Drawing for the job (mm, zero at the part's lowest x, y, z). A direction names the side the tool comes from. Give positions to 0.01 mm unless a question says otherwise; leave off trailing zeros. Loops run counter-clockwise (first coordinate to the right, second up) from the corner with the lowest first, then second, coordinate; pieces in that order, holes last. Notation, with made-up numbers: M 83.5,13 L 89.5,13 A17 ccw 89.5,22 Z; hole C 31.25,10.5 d5. An arc over 180 degrees is marked long. Use CSV: the item, a comma, the result in double quotes. Start each with the question number.
(1) Tool access for the marked faces 1, 2 and 3: list every direction of +Z, -Z, +X, -X, +Y, -Y with a clear straight run to the whole face (end or side of a thin tool).
(2) Slice it at A-A on y = 11. List the corners of the cut face in (x, z).
(3) Two-plate mould, pull along Y, no slides. Class the marked faces 4, 5 and 6: pulls with the +Y half, pulls with the -Y half, needs draft (parallel to the pull), parting line crosses it, or undercut.
(4) Slice it at D-D on y = 19.5. List the corners of the cut face in (x, z).
(5) Slice it at B-B on z = 14.5. List the corners of the cut face in (x, y).
(6) Wall check: line 1 along Y through (x, z) = (13.5, 12.25); line 2 along Y through (x, z) = (9, 11.25) (1 decimal); line 3 along X through (y, z) = (13, 15). Give the ranges that are in metal, low to high. Write a range as from..to.
(7) Slice it at C-C on x = 15. List the corners of the cut face in (y, z).
(8) Flat gauge pins, fed straight in: P1, Ø1, axis at x = 24, y = 22.5, coming from the -Z side; P2, Ø4, axis at x = 12.5, y = 15.5, coming from the +Z side; P3, Ø6, axis at x = 13.5, z = 16, coming from the -Y side. Where does each tip first touch, or does it go through?
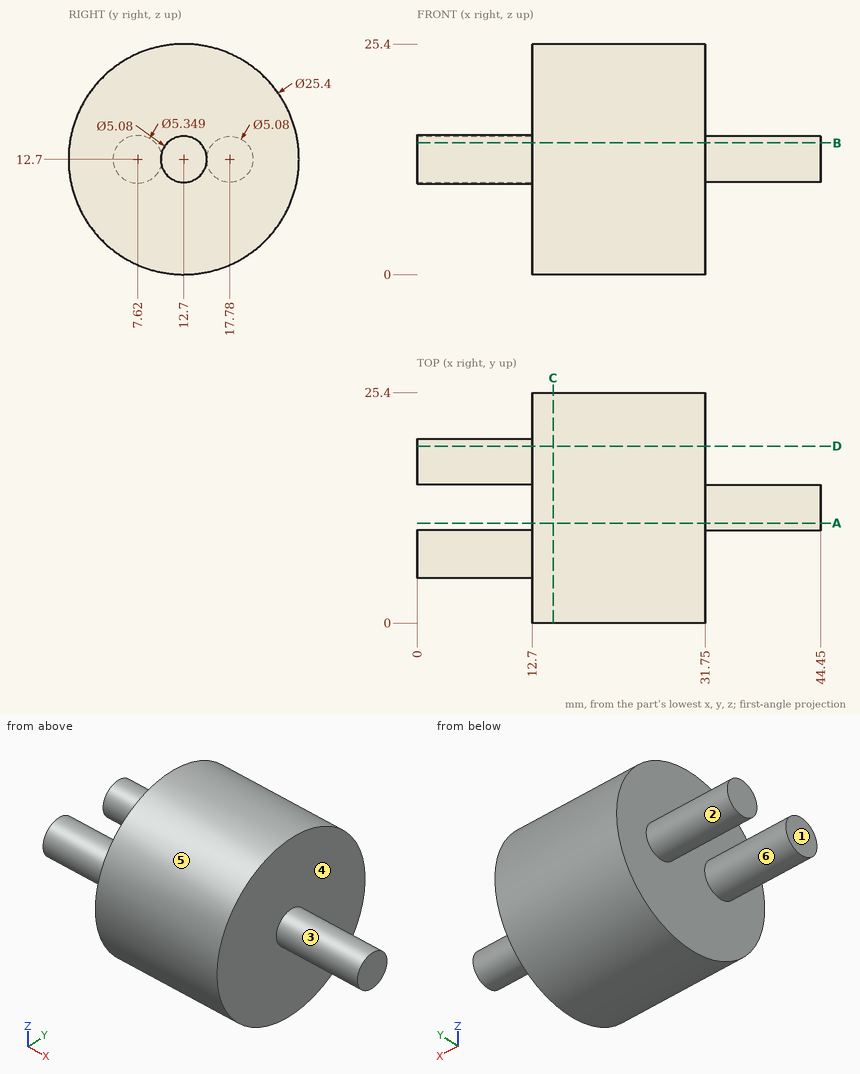
Reply:
1,face 1,"+Z, -Z, -X, +Y, -Y"
1,face 2,"-X"
1,face 3,"+X"
2,outline,"M 12.7,0.11 L 31.75,0.11 L 31.75,10.81 L 44.45,10.81 L 44.45,14.59 L 31.75,14.59 L 31.75,25.29 L 12.7,25.29 Z"
3,face 4,"needs draft"
3,face 5,"parting line crosses it"
3,face 6,"undercut"
4,outline,"M 0,10.83 L 12.7,10.83 L 12.7,1.97 L 31.75,1.97 L 31.75,23.43 L 12.7,23.43 L 12.7,14.57 L 0,14.57 Z"
5,outline,"M 0,5.64 L 12.7,5.64 L 12.7,0.13 L 31.75,0.13 L 31.75,10.91 L 44.45,10.91 L 44.45,14.49 L 31.75,14.49 L 31.75,25.27 L 12.7,25.27 L 12.7,19.57 L 0,19.57 L 0,15.99 L 12.7,15.99 L 12.7,9.6 L 0,9.6 Z"
6,line 1,"y = 0.01..25.39"
6,line 2,"y = 5.4..9.9, 15.7..19.9"
6,line 3,"x = 12.7..44.45"
7,outline,"C 12.7,12.7 d25.4"
8,P1,"stops at z = 4.05"
8,P2,"stops at z = 25.37"
8,P3,"stops at y = 0"
